Work out the finished part from the listing and answer in its coordinate system (mm). A direction names the side the tool comes from. Round coordinates to 2 decimals unless told otherwise and drop trailing zeros. Loops run counter-clockwise (first coordinate to the right, second up) from the corner with the lowest first, then second, coordinate; pieces in that order, holes last.
from build123d import *

# Parameters (mm, degrees)
F1_DEPTH = 76.2
F3_DEPTH = 76.201
F4_R     = 19.05
F4_R_2   = 6.35
F5_DEPTH = 12.7
F6_DEPTH = 76.201


with BuildPart() as f1:
    # F0 (on Front) → F1 (new body)
    with BuildSketch(Plane.XZ):
        Polygon((0, 127), (0, 0), (177.8, 0), (177.8, 28.575), (101.6, 28.575), (101.6, 127), align=None)
    extrude(amount=F1_DEPTH)

    # F2 (on face) → F3 (cut, through all)
    with BuildSketch(Plane.XZ.offset(76.2)):
        with BuildLine():
            Line((0, 127), (0, 76.2))
            ThreePointArc((0, 76.2), (14.4878771466, 111.7306783097), (49.6898018168, 127))
            Line((49.6898018168, 127), (0, 127))
        make_face()
        with BuildLine():
            Line((101.6, 127), (51.9350028707, 127))
            ThreePointArc((51.9350028707, 127), (86.5773951149, 112.2938432981), (101.6, 77.7875))
            Line((101.6, 77.7875), (101.6, 127))
        make_face()
    extrude(amount=-F3_DEPTH, mode=Mode.SUBTRACT)

    # F4 (on face) → F5 (cut)
    with BuildSketch(Plane.XZ.offset(76.2)):
        with Locations((50.8, 76.2)):
            Circle(F4_R)
        with Locations((50.8, 76.2)):
            Circle(F4_R_2, mode=Mode.SUBTRACT)
    extrude(amount=-F5_DEPTH, mode=Mode.SUBTRACT)

    # F6 (cut, through all): a face of the model
    f6_faces = [f1.faces().sort_by_distance(p)[0] for p in [
        (50.8, -76.2, 76.2),
    ]]
    extrude(f6_faces, amount=-F6_DEPTH, mode=Mode.SUBTRACT)


solid = f1.part
Item 1: Section B-B, the plane z = 88.5 is taken. Give the vertices of the cut face in (x, y).
Item 2: Straight lines are drawn through the part: line 1 (Z direction, x = 50.8, y = -67.25); line 2 (Z direction, x = 50.8, y = -16.5); line 3 (Z direction, x = 136, y = -14.5) (3 decimals). For each, find the intervals that lie inside material, in ascending order.
Item 3: Section D-D, the plane x = 80 is taken. Give the vertices of the cut face in (y, z).
Item 4: Section C-C, the plane x = 110 is taken. Give the vertices of the cut face in (y, z) (3 decimals), plus the area to 3 significant figures.
Item 5: Each of these flat-tipped pins is pushed along its axis until it touches: P1, Ø2, axis at y = -9.5, z = 44, coming from the +X side; P2, Ø3, axis at x = 61.5, z = 94, coming from the +Y side; P3, Ø6, axis at x = 32.5, y = -25, coming from the +Z side; P4, Ø5, axis at x = 33.5, y = -9, coming from the +Z side. Where does it stop, or does it pass through?
Item 6: For faces 1 (the face through (177.8, -38, 14)), 2 (the face through (140, -38, 28.575)), 3 (the face through (46, -63.5, 81)), determine the directions among +Z, -Z, +X, -X, +Y, -Y from which every point of the face is accessible in a straight line to the end or side of a thin tool.
Item 7: Determine the mould class of faces 4 (the face through (101.6, -38, 53)), 5 (the face through (36.759, -69.939, 89.075)), 6 (the face through (14.1, -38.63, 111.33)) for opening direction X: pulls with the +X half, pulls with the -X half, needs draft (parallel to the pull), parting line crosses it, or undercut.
Answer below:
1. outline: (1.51, -76.2) - (36.25, -76.2) - (36.25, -63.5) - (65.35, -63.5) - (65.35, -76.2) - (100.11, -76.2) - (100.11, 0) - (1.51, 0) - close
2. line 1: z = 0 to 57.15, 95.25 to 127
2. line 2: z = 0 to 69.85, 82.55 to 127
2. line 3: z = 0 to 28.575
3. outline: (-76.2, 0) - (0, 0) - (0, 117.79) - (-76.2, 117.79) - close
4. outline: (-76.2, 0) - (0, 0) - (0, 28.575) - (-76.2, 28.575) - close
4. area: 2,180 mm2
5. P1: stops at x = 101.6
5. P2: stops at y = 0
5. P3: stops at z = 124.65
5. P4: stops at z = 124.81
6. face 1: +Z, -Z, +X, +Y, -Y
6. face 2: +Z, +X, +Y, -Y
6. face 3: -Y
7. face 4: pulls with the +X half
7. face 5: undercut
7. face 6: pulls with the -X half
